Geometry check sheet. Reference: the model listing, model coordinates, mm. A direction names the side the tool comes from. Coordinates: 2 decimals unless noted, no trailing zeros. Write each loop counter-clockwise with the first axis right and the second up, starting at its lowest first coordinate (ties: lowest second). Pieces come first, ordered by that corner, then holes. Notation, with made-up numbers: M 60.5,87.5 L 94.5,87.5 A22 ccw 94.5,100.5 Z; hole C 76,5.25 d1. An arc over 180 degrees is marked long. Write item = value, one per line. Start each with the question number.
```python
from build123d import *

# Parameters (mm, degrees)
BOSS_EXTRUDE1_OUTLINE_R = 3.556
BOSS_EXTRUDE1_OUTLINE_W = 260.9469
BOSS_EXTRUDE1_OUTLINE_H = 138.1252
BOSS_EXTRUDE1_DEPTH     = 76.2
CUT_EXTRUDE1_DEPTH      = 355.32482824
CUT_EXTRUDE1_DEPTH_BACK = 355.32482824
FILLET1_R               = 2.54
SKETCH7_W               = 260.9469
SKETCH7_H               = 22.1996
CUT_EXTRUDE2_DEPTH      = 347.152897849
FILLET2_R               = 6.35
SKETCH8_W               = 217.439036591
SKETCH8_H               = 235.521960295
CUT_EXTRUDE4_DEPTH      = 347.144751077
SKETCH9_W               = 205.813387363
SKETCH9_H               = 113.418104201
CUT_EXTRUDE5_DEPTH      = 347.144751077


# Read off the part's stored shape, not the designer's step: Boss-Extrude1
with BuildPart() as part:
    # Boss-Extrude1 outline → Boss-Extrude1 (new body)
    with BuildSketch(Plane.XY):
        with BuildLine():
            Line((-286.3596, -22.225), (9.525, -22.225))
            ThreePointArc((9.525, -22.225), (19.05, -12.7), (9.525, -3.175))
            ThreePointArc((9.525, -3.175), (19.05, 6.35), (9.525, 15.875))
            ThreePointArc((9.525, 15.875), (2.789807909, 18.664807909), (0, 25.4))
            Line((0, 25.4), (0, 131.7752))
            ThreePointArc((0, 131.7752), (2.789807909, 138.510392091), (9.525, 141.3002))
            ThreePointArc((9.525, 141.3002), (19.05, 150.8252), (9.525, 160.3502))
            ThreePointArc((9.525, 160.3502), (19.05, 169.8752), (9.525, 179.4002))
            Line((9.525, 179.4002), (-6.35, 179.4002))
            Line((-6.35, 179.4002), (-6.35, 163.5252))
            Line((-6.35, 163.5252), (-7.9502, 163.5252))
            Line((-7.9502, 163.5252), (-7.9502, 160.3502))
            Line((-7.9502, 160.3502), (-268.9098, 160.3502))
            Line((-268.9098, 160.3502), (-268.9098, 163.5252))
            Line((-268.9098, 163.5252), (-270.51, 163.5252))
            Line((-270.51, 163.5252), (-270.51, 179.4002))
            Line((-270.51, 179.4002), (-286.385, 179.4002))
            ThreePointArc((-286.385, 179.4002), (-295.91, 169.8752), (-286.385, 160.3502))
            ThreePointArc((-286.385, 160.3502), (-295.897297883, 150.818850004), (-286.3723, 141.3002))
            ThreePointArc((-286.3723, 141.3002), (-279.637107909, 138.510392091), (-276.8473, 131.7752))
            Line((-276.8473, 131.7752), (-276.8473, 25.4))
            ThreePointArc((-276.8473, 25.4), (-279.637107909, 18.664807909), (-286.3723, 15.875))
            ThreePointArc((-286.3723, 15.875), (-295.8973, 6.35), (-286.3723, -3.175))
            ThreePointArc((-286.3723, -3.175), (-295.884597883, -12.706349996), (-286.3596, -22.225))
        make_face()
        with Locations((-286.3596, -12.7)):
            Circle(BOSS_EXTRUDE1_OUTLINE_R, mode=Mode.SUBTRACT)
        with Locations((-286.3723, 6.35)):
            Circle(BOSS_EXTRUDE1_OUTLINE_R, mode=Mode.SUBTRACT)
        with Locations((9.525, -12.7)):
            Circle(BOSS_EXTRUDE1_OUTLINE_R, mode=Mode.SUBTRACT)
        with Locations((9.525, 6.35)):
            Circle(BOSS_EXTRUDE1_OUTLINE_R, mode=Mode.SUBTRACT)
        with Locations((-286.3723, 150.8252)):
            Circle(BOSS_EXTRUDE1_OUTLINE_R, mode=Mode.SUBTRACT)
        with Locations((-286.385, 169.8752)):
            Circle(BOSS_EXTRUDE1_OUTLINE_R, mode=Mode.SUBTRACT)
        with Locations((-138.42365, 78.5876)):
            Rectangle(BOSS_EXTRUDE1_OUTLINE_W, BOSS_EXTRUDE1_OUTLINE_H, mode=Mode.SUBTRACT)
        with Locations((9.525, 150.8252)):
            Circle(BOSS_EXTRUDE1_OUTLINE_R, mode=Mode.SUBTRACT)
        with Locations((9.525, 169.8752)):
            Circle(BOSS_EXTRUDE1_OUTLINE_R, mode=Mode.SUBTRACT)
    extrude(amount=BOSS_EXTRUDE1_DEPTH)

    # Sketch5 → Cut-Extrude1 (cut, two sides: drawn at the far end of the back side and taken through both)
    with BuildSketch(Plane.ZY.offset(276.8473).offset(-CUT_EXTRUDE1_DEPTH_BACK)):
        Polygon((1.6002, -22.225), (8.641107133, 179.4002), (76.2, 179.4002), (76.2, -22.225), align=None)
    extrude(amount=CUT_EXTRUDE1_DEPTH + CUT_EXTRUDE1_DEPTH_BACK, mode=Mode.SUBTRACT)

    # Fillet1
    fillet1_edges = [part.edges().sort_by_distance(p)[0] for p in [
        (-286.385, 160.3502, 3.987933237),
        (-286.3723, -3.175, 1.132720329),
        (9.525, -3.175, 1.132720329),
        (9.525, 160.3502, 3.987933237),
    ]]
    fillet(fillet1_edges, radius=FILLET1_R)

    # Sketch7 → Cut-Extrude2 (cut, through all)
    with BuildSketch(Plane(origin=(0, 0, 0), x_dir=(-1, 0, 0), z_dir=(0, 0, -1))):
        with Locations((138.42365, -6.35)):
            Rectangle(SKETCH7_W, SKETCH7_H)
    extrude(amount=-CUT_EXTRUDE2_DEPTH, mode=Mode.SUBTRACT)

    # Fillet2
    fillet2_edges = [part.edges().sort_by_distance(p)[0] for p in [
        (-268.8971, 4.7498, 1.271090386),
        (-268.8971, -17.4498, 0.883476829),
        (-7.9502, -17.4498, 0.883476829),
        (-7.9502, 4.7498, 1.271090386),
    ]]
    fillet(fillet2_edges, radius=FILLET2_R)

    # Sketch8 → Cut-Extrude4 (cut, through all)
    with BuildSketch(Plane(origin=(0, -0.082881646, 2.373419811), x_dir=(1, 0, 0), z_dir=(0, -0.03489949670250444, 0.9993908270190958))):
        with Locations((-29.704131704, 74.917246318)):
            Rectangle(SKETCH8_W, SKETCH8_H)
    extrude(amount=-CUT_EXTRUDE4_DEPTH, mode=Mode.SUBTRACT)

    # Sketch9 → Cut-Extrude5 (cut, through all)
    with BuildSketch(Plane(origin=(0, -0.082881646, 2.373419811), x_dir=(1, 0, 0), z_dir=(0, -0.03489949670250444, 0.9993908270190958))):
        with Locations((-241.330343682, 135.427486891)):
            Rectangle(SKETCH9_W, SKETCH9_H)
    extrude(amount=-CUT_EXTRUDE5_DEPTH, mode=Mode.SUBTRACT)


solid = part.part
```
Q1. Scan lines: L1, parallel to Y at x = -186, z = 1.2 (3 decimals); L2, parallel to X at y = 6.35, z = 1.15; L3, parallel to X at y = -12.7, z = 1. Record each from-to range of solid material in increasing order.
Q2. Cross-section at B-B on y = -12.7. Enter the section's corners in (x, z).
Q3. Cross-section at C-C on y = 12.5. Enter the section's corners in (x, z).
Q4. Set-up check for faces 1 (the face through (-268.897, 44, 2)), 2 (the face through (-266.988, 2.939, 1.289)), 3 (the face through (-295.42, -15.64, 0.84)): record each of +Z, -Z, +X, -X, +Y, -Y from which the full face is reachable in a straight line by a thin tool's end or side.
Q5. Gauge pin test, flat ends, axial feed: pin 1 (1.9 mm diameter, centred on y = -6, z = 1, fed in from +X); pin 2 (0.9 mm diameter, centred on x = -193, z = 1, fed in from +Y) (3 decimals). Record the tip position at first contact, or that the pin passes through.
Q6. Cross-section at A-A on x = -221.5. Enter the section's corners in (y, z) (3 decimals), and give its area (3 significant figures).
Q7. Cross-section at D-D on x = -280. Enter the section's corners in (y, z) (1 decimal), and give its area (3 significant figures).
Q8. Draft check along Y on faces 4 (the face through (-276.847, 52, 2)), 5 (the face through (-267.086, -15.54, 1.008)). Enter one of: pulls with the +Y half, pulls with the -Y half, needs draft (parallel to the pull), parting line crosses it, or undercut.
Values found:
q1.L1 = -22.225 to -17.45, 4.75 to 9.525
q1.L2 = -295.9 to -289.93, -282.82 to -138.42
q1.L3 = -295.88 to -289.92, -282.8 to -268.69
q2.outline = M -295.88,0 L -289.92,0 L -289.92,1.93 L -295.88,1.93 Z; M -282.8,0 L -268.69,0 L -268.69,1.93 L -282.8,1.93 Z
q3.outline = M -293.65,0 L -268.9,0 L -268.9,2.81 L -293.65,2.81 Z
q4.face_1 = +Z, -Z, +X, +Y
q4.face_2 = +Z, -Z, +X
q4.face_3 = +Z, -Z, -X
q5.pin_1 = -268.9
q5.pin_2 = 9.525
q6.outline = M -22.225,0 L -17.45,0 L -17.45,1.767 L -22.225,1.6 Z; M 4.75,0 L 9.525,0 L 9.525,2.709 L 4.75,2.542 Z
q6.area = 20.6 mm²
q7.outline = M -22.2,0 L 18.3,0 L 18.3,3 L -22.2,1.6 Z
q7.area = 93.6 mm²
q8.face_4 = needs draft
q8.face_5 = undercut
